The model under review builds one solid part; all positions refer to its coordinate system, in mm. Round coordinates to 2 decimals unless told otherwise and drop trailing zeros. Write each loop counter-clockwise with the first axis right and the second up, starting at its lowest first coordinate (ties: lowest second). Pieces come first, ordered by that corner, then holes. Notation, with made-up numbers: (-9, 76.25) - (43, 76.25) arc R14 cw to (43, 89.25) - close; hole circle Ø2 at (-9, 29.25). An arc over 180 degrees is marked (long way). Write each question's results on one line, items separated by ' | '.
```python
from build123d import *

# Parameters (mm, degrees)
SKETCH_1_R      = 2
SKETCH_1_R_2    = 5.02
SKETCH_1_R_3    = 2.05
SKETCH_1_W      = 8.2
SKETCH_1_H      = 2.2
EXTRUDE_1_DEPTH = 2
FILLET_1_R      = 1


with BuildPart() as part:
    # 草图1 → 凸台-拉伸1 (new body)
    with BuildSketch(Plane.XY):
        with BuildLine():
            Line((-38.25, 66.25), (-38.25, 62.25))
            Line((-38.25, 62.25), (-40.15, 62.25))
            Line((-40.15, 62.25), (-40.15, 59.05))
            Line((-40.15, 59.05), (-38.25, 59.05))
            Line((-38.25, 59.05), (-38.25, 55.85))
            Line((-38.25, 55.85), (-34.15, 55.85))
            Line((-34.15, 55.85), (-34.15, 59.05))
            Line((-34.15, 59.05), (-32.25, 59.05))
            Line((-32.25, 59.05), (-32.25, 62.25))
            Line((-32.25, 62.25), (-34.15, 62.25))
            Line((-34.15, 62.25), (-34.15, 66.25))
            Line((-34.15, 66.25), (-25.2, 66.25))
            Line((-25.2, 66.25), (-25.2, 70.25))
            Line((-25.2, 70.25), (-17.2, 70.25))
            Line((-17.2, 70.25), (-17.2, 66.25))
            Line((-17.2, 66.25), (-8.25, 66.25))
            Line((-8.25, 66.25), (-8.25, 62.25))
            Line((-8.25, 62.25), (-10.15, 62.25))
            Line((-10.15, 62.25), (-10.15, 59.05))
            Line((-10.15, 59.05), (-8.25, 59.05))
            Line((-8.25, 59.05), (-8.25, 55.85))
            Line((-8.25, 55.85), (-4.15, 55.85))
            Line((-4.15, 55.85), (-4.15, 59.05))
            Line((-4.15, 59.05), (-2.25, 59.05))
            Line((-2.25, 59.05), (-2.25, 62.25))
            Line((-2.25, 62.25), (-4.15, 62.25))
            Line((-4.15, 62.25), (-4.15, 66.25))
            Line((-4.15, 66.25), (4.8, 66.25))
            Line((4.8, 66.25), (4.8, 57.55))
            Line((4.8, 57.55), (53.96460577, -41.768082641))
            ThreePointArc((53.96460577, -41.768082641), (38.925737517, -73.658373169), (11.3, -51.75))
            Line((11.3, -51.75), (-94.15, 57.55))
            Line((-94.15, 57.55), (-94.15, 66.25))
            Line((-94.15, 66.25), (-85.2, 66.25))
            Line((-85.2, 66.25), (-85.2, 70.25))
            Line((-85.2, 70.25), (-77.2, 70.25))
            Line((-77.2, 70.25), (-77.2, 66.25))
            Line((-77.2, 66.25), (-68.25, 66.25))
            Line((-68.25, 66.25), (-68.25, 62.25))
            Line((-68.25, 62.25), (-70.15, 62.25))
            Line((-70.15, 62.25), (-70.15, 59.05))
            Line((-70.15, 59.05), (-68.25, 59.05))
            Line((-68.25, 59.05), (-68.25, 55.85))
            Line((-68.25, 55.85), (-64.15, 55.85))
            Line((-64.15, 55.85), (-64.15, 59.05))
            Line((-64.15, 59.05), (-62.25, 59.05))
            Line((-62.25, 59.05), (-62.25, 62.25))
            Line((-62.25, 62.25), (-64.15, 62.25))
            Line((-64.15, 62.25), (-64.15, 66.25))
            Line((-64.15, 66.25), (-55.2, 66.25))
            Line((-55.2, 66.25), (-55.2, 70.25))
            Line((-55.2, 70.25), (-47.2, 70.25))
            Line((-47.2, 70.25), (-47.2, 66.25))
            Line((-47.2, 66.25), (-38.25, 66.25))
        make_face()
        with Locations((-19.762745434, 31.422010331)):
            Circle(SKETCH_1_R, mode=Mode.SUBTRACT)
        with Locations((7.098407643, -10.75)):
            Circle(SKETCH_1_R, mode=Mode.SUBTRACT)
        with Locations((33.85, -52.75)):
            Circle(SKETCH_1_R_2, mode=Mode.SUBTRACT)
        with Locations((-6.332168895, 10.336005166)):
            Circle(SKETCH_1_R_3, mode=Mode.SUBTRACT)
        with Locations((-7.901592357, -10.75)):
            Rectangle(SKETCH_1_W, SKETCH_1_H, mode=Mode.SUBTRACT)
    extrude(amount=EXTRUDE_1_DEPTH)

    # 圆角1
    fillet_1_edges = [part.edges().sort_by_distance(p)[0] for p in [
        (-25.2, 70.25, 1),
        (-17.2, 70.25, 1),
        (-85.2, 70.25, 1),
        (-77.2, 70.25, 1),
        (-55.2, 70.25, 1),
        (-47.2, 70.25, 1),
    ]]
    fillet(fillet_1_edges, radius=FILLET_1_R)


solid = part.part
```
Q1. We need section C-C (z = 0.6). State how many separate pieces and enclosed holes the cut face has, plus the area to 3 significant figures.
Evaluation:
separate pieces: 1 | enclosed holes: 5 | area: 9,450 mm^2
Q2. We need section D-D (x = -30). State the section outline as (y, z) points.
Evaluation:
outline: (-8.94, 0) - (66.25, 0) - (66.25, 2) - (-8.94, 2) - close
Q3. We need section B-B (x = -82). State the section outline as (y, z) points.
Evaluation:
outline: (44.96, 0) - (70.25, 0) - (70.25, 2) - (44.96, 2) - close
Q4. For probe 1 along X at (y, z) = (59, 0.3); probe 2 along X at (y, z) = (-10, 1.5); probe 3 along X at (y, z) = (-52.5, 0.45), list the stretches that pass through material, from the lowest coordinate up.
Evaluation:
probe 1: x = -94.15 to -68.25, -64.15 to -38.25, -34.15 to -8.25, -4.15 to 4.8 | probe 2: x = -28.98 to -12, -3.8 to 5.24, 8.95 to 38.24 | probe 3: x = 11.31 to 28.84, 38.86 to 56.29
Q5. The part is to be moulded in two halves that separate along Y. For faces 1 (the flat face through (-40.687, 2.135, 0.986)), 2 (the cylindrical face through (-6.6, 12.37, 0.99)), 3 (the flat face through (-1, 15, 2)), 4 (the cylindrical face through (9.006, -10.149, 0.986)), say which applies: released by +Y, released by -Y, zero draft, split by the parting line, or undercut.
Evaluation:
face 1: released by -Y | face 2: undercut | face 3: zero draft | face 4: undercut
Q6. We need section A-A (x = 33.85). State the section outline as (y, z) points, plus the area to 3 significant figures.
Evaluation:
outline: (-74.25, 0) - (-57.77, 0) - (-57.77, 2) - (-74.25, 2) - close; (-47.73, 0) - (-1.13, 0) - (-1.13, 2) - (-47.73, 2) - close | area: 126 mm^2
Q7. Insertion check: P1, Ø1, axis at y = 39, z = 1, coming from the +X side; P2, Ø1, axis at y = 68, z = 0.5, coming from the +X side; P3, Ø0.6, axis at y = 64.5, z = 1, coming from the +X side; P4, Ø5, axis at x = 7.1, y = -10.75, coming from the +Z side. Each pin has a flat end and moves straight along its axis. Give the tip position at first contact, or say it passes through.
Evaluation:
P1: stops at x = 14.23 | P2: stops at x = -17.2 | P3: stops at x = 4.8 | P4: stops at z = 2
